from build123d import *

# Parameters (mm, degrees)
BOSS_EXTRUDE1_DEPTH             = 3
TAP_DRILL_FOR_M3X0_5_TAP1_D     = 2.5
TAP_DRILL_FOR_M3X0_5_TAP1_DEPTH = 3


with BuildPart() as part:
    # Sketch1 → Boss-Extrude1 (new body)
    with BuildSketch(Plane(origin=(0, 0, 0), x_dir=(0, 0, -1), z_dir=(1, 0, 0))):
        Polygon((0, 0), (0, 35), (3.3, 35), (3.3, 19), (8, 19), (8, 0), align=None)
    extrude(amount=BOSS_EXTRUDE1_DEPTH)

    # Tap Drill for M3x0.5 Tap1
    with Locations(Plane(origin=(3, 0, 0), x_dir=(0, 0, -1), z_dir=(1, 0, 0))):
        with Locations((5, 15.4), (5, 3.4)):
            Hole(TAP_DRILL_FOR_M3X0_5_TAP1_D / 2, depth=TAP_DRILL_FOR_M3X0_5_TAP1_DEPTH)


solid = part.part
Source: CAD feature listing. Evaluate the final solid. Frame: model axes, mm. A direction names the side the tool comes from. Give positions to 0.01 mm unless a question says otherwise; leave off trailing zeros. Order: outer loops, then holes, each group sorted by start corner. A loop starts at its lowest first (then second) coordinate and runs counter-clockwise, first axis right, second up. Notation, with made-up numbers: (-38, 39) -> (16, 39) arc R17 ccw to (16, 51) -> close; hole circle Ø5 at (-22.75, -11). An arc over 180 degrees is marked (long way). Use a Markdown table: item, result.
1) Ray query, line 1 along Y through (x, z) = (1.7, -5); line 2 along Y through (x, z) = (2.4, -6); line 3 along Z through (x, y) = (0.75, 31.5). Return the intervals inside material, ascending. Write a range as [from, to].
Answer list:
| item | result |
|---|---|
| line 1 | [0, 2.15], [4.65, 14.15], [16.65, 19] |
| line 2 | [0, 2.65], [4.15, 14.65], [16.15, 19] |
| line 3 | [-3.3, 0] |
2) Contact query for a flat-ended pin moving along its axis: P1, Ø0.9, axis at x = 2, z = -6, coming from the +Y side. Output: stop coordinate, or through.
Answer list:
| item | result |
|---|---|
| P1 | y = 19 |
3) Section query C-C, the plane x = 1.35. Return the cut outline in (y, z), then the cut area to 3 significant figures.
Answer list:
| item | result |
|---|---|
| outline | (0, -8) -> (19, -8) -> (19, -3.3) -> (35, -3.3) -> (35, 0) -> (0, 0) -> close; hole circle Ø2.5 at (3.4, -5); hole circle Ø2.5 at (15.4, -5) |
| area | 195 mm² |
4) Mould query, pull axis Z, two halves, no side actions, for faces 1 (the cylindrical face through (1.48, 14.18, -5.27)), 2 (the flat face through (1, 19, -6)), 3 (the flat face through (1, 10, -8)). Classes: +Z half, -Z half, draft (parallel to the pull), parting line (faces both ways), or undercut.
Answer list:
| item | result |
|---|---|
| face 1 | undercut |
| face 2 | draft |
| face 3 | -Z half |
5) Reachability of faces 4 (the flat face through (1, 35, -2)), 5 (the flat face through (1, 27, -3.3)) from +Z, -Z, +X, -X, +Y, -Y: full face, straight path, thin tool, end or side. Return the list, or none.
Answer list:
| item | result |
|---|---|
| face 4 | +Z, -Z, +X, -X, +Y |
| face 5 | -Z, +X, -X, +Y |
6) Section query A-A, the plane z = -5. Return the cut outline in (x, y).
Answer list:
| item | result |
|---|---|
| outline | (0, 0) -> (3, 0) -> (3, 2.15) -> (0, 2.15) -> close; (0, 4.65) -> (3, 4.65) -> (3, 14.15) -> (0, 14.15) -> close; (0, 16.65) -> (3, 16.65) -> (3, 19) -> (0, 19) -> close |
7) Section query D-D, the plane y = 30.5. Return the cut outline in (x, z).
Answer list:
| item | result |
|---|---|
| outline | (0, -3.3) -> (3, -3.3) -> (3, 0) -> (0, 0) -> close |
8) Section query B-B, the plane y = 15.4. Return the cut outline in (x, z), then the cut area to 3 significant figures.
Answer list:
| item | result |
|---|---|
| outline | (0, -8) -> (3, -8) -> (3, -6.25) -> (0, -6.25) -> close; (0, -3.75) -> (3, -3.75) -> (3, 0) -> (0, 0) -> close |
| area | 16.5 mm² |
